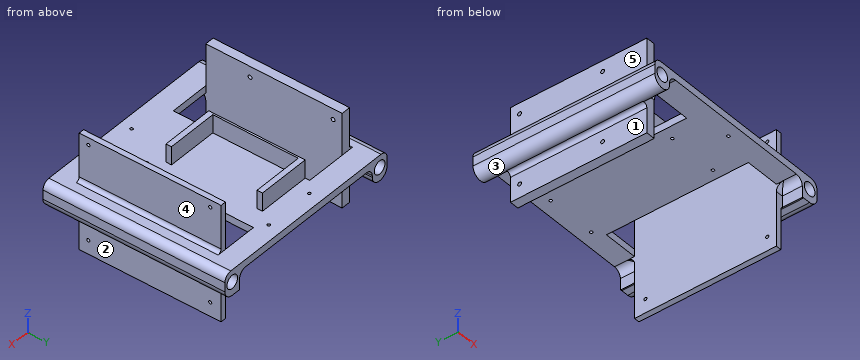
```python
from build123d import *

# Parameters (mm, degrees)
BOSS_EXTRUDE1_DEPTH      = 127
SKETCH3_R                = 4.60374999999995
SKETCH3_R_2              = 4.603749999999996
CUT_EXTRUDE1_DEPTH       = 127
CUT_EXTRUDE10_DEPTH      = 190.225738207042
CUT_EXTRUDE10_DEPTH_BACK = 190.225738207042
SKETCH19_W               = 27.939999999999998
SKETCH19_H               = 99.05999999999997
BOSS_EXTRUDE6_DEPTH      = 3.8099999999999996
CUT_EXTRUDE11_DEPTH      = 183.54455346572246
CUT_EXTRUDE11_DEPTH_BACK = 183.54455346572246
SKETCH23_R               = 1.0999978000000017
SKETCH23_R_2             = 1.0999978000000061
SKETCH23_R_3             = 1.099997799999995
BOSS_EXTRUDE8_DEPTH      = 31.75
BOSS_EXTRUDE8_DEPTH_BACK = 34.29
CUT_EXTRUDE12_DEPTH      = 194.67395901359583
CUT_EXTRUDE12_DEPTH_BACK = 194.67395901359583
CUT_EXTRUDE13_DEPTH      = 194.67395901359583
CUT_EXTRUDE13_DEPTH_BACK = 194.67395901359583
SKETCH32_R               = 0.9999980000000093
SKETCH34_R               = 1.3499972999999863
SKETCH34_R_2             = 1.349997299999995
SKETCH34_R_3             = 1.3499973000000016
CUT_EXTRUDE15_DEPTH      = 15.239999999999998
BOSS_EXTRUDE10_DEPTH     = 12.7
SKETCH36_W               = 1.2700000000000102
SKETCH36_H               = 12.700000000000014
BOSS_EXTRUDE11_DEPTH     = 99.06
FILLET5_R                = 2.54
FILLET6_R                = 2.54
FILLET7_R                = 5.08


with BuildPart() as part:
    # Sketch2 → Boss-Extrude1 (new body)
    with BuildSketch(Plane(origin=(0, 0, 0), x_dir=(1, 0, 0), z_dir=(0, 1, 0))):
        with BuildLine():
            Line((8.7e-16, 11.429999999999996), (8.7e-16, 5.079999999999999))
            ThreePointArc((8.7e-16, 5.079999999999999), (1.4878975515723396, 1.4878975515723383), (5.080000000000001, 0))
            Line((5.080000000000001, 0), (134.61999999999998, 0))
            ThreePointArc((134.61999999999998, 0), (138.21210244842763, 1.4878975515723387), (139.7, 5.08))
            Line((139.7, 5.08), (139.70000000000002, 11.429999999999996))
            ThreePointArc((139.70000000000002, 11.429999999999996), (137.8401280605346, 15.920128060534589), (133.35, 17.78000000000002))
            Line((133.35, 17.78000000000002), (127, 17.780000000000015))
            Line((127, 17.780000000000015), (127, 11.429999999999996))
            Line((127, 11.429999999999996), (127, 5.079999999999999))
            Line((127, 5.079999999999999), (12.699999999999989, 5.08))
            Line((12.699999999999989, 5.08), (12.699999999999989, 11.429999999999996))
            ThreePointArc((12.699999999999989, 11.429999999999996), (6.349999999999994, 17.77999999999999), (8.7e-16, 11.429999999999996))
        make_face()
    extrude(amount=BOSS_EXTRUDE1_DEPTH)

    # Sketch3 → Cut-Extrude1 (cut)
    with BuildSketch(Plane(origin=(0, 127, 0), x_dir=(1, 0, 0), z_dir=(0, 1, 0))):
        with Locations(Location((133.35, 8.41375, 0), (0, 0, 270))):
            Circle(SKETCH3_R)
        with Locations(Location((6.349999999999994, 8.41375, 0), (0, 0, 270))):
            Circle(SKETCH3_R_2)
    extrude(amount=-CUT_EXTRUDE1_DEPTH, mode=Mode.SUBTRACT)

    # Sketch19 → Cut-Extrude10 (cut, two sides: drawn at the far end of the back side and taken through both)
    with BuildSketch(Plane(origin=(4e-17, 0, -5.08), x_dir=(-1, 0, -1e-17), z_dir=(1e-17, 0, -1)).offset(-CUT_EXTRUDE10_DEPTH_BACK)):
        with Locations((-111.76, 63.5)):
            Rectangle(SKETCH19_W, SKETCH19_H)
    extrude(amount=CUT_EXTRUDE10_DEPTH + CUT_EXTRUDE10_DEPTH_BACK, mode=Mode.SUBTRACT)

    # Sketch20 → Boss-Extrude6 (add)
    with BuildSketch(Plane(origin=(125.73, 0, 9.5e-16), x_dir=(1e-17, 0, -1), z_dir=(1, 0, 1e-17))):
        Polygon((5.08, 113.02999999999999), (48.26, 113.02999999999999), (48.26000000000001, 13.97000000000001), (5.08, 13.97000000000001), (-1.06e-15, 13.97000000000001), (-33.01999999999999, 13.97000000000001), (-33.02, 113.02999999999999), (-1.06e-15, 113.02999999999999), align=None)
    extrude(amount=-BOSS_EXTRUDE6_DEPTH)

    # Sketch23 → Cut-Extrude11 (cut, two sides: drawn at the far end of the back side and taken through both)
    with BuildSketch(Plane.ZY.offset(-121.92000000000002).offset(-CUT_EXTRUDE11_DEPTH_BACK)):
        with Locations((27.94, 105.45831715747836)):
            Circle(SKETCH23_R)
        with Locations((27.94, 20.32000000000001)):
            Circle(SKETCH23_R_2)
        with Locations((-38.55999400000001, 20.32000000000001)):
            Circle(SKETCH23_R_3)
        with Locations((-38.55999400000001, 105.45831715747836)):
            Circle(SKETCH23_R_3)
    extrude(amount=CUT_EXTRUDE11_DEPTH + CUT_EXTRUDE11_DEPTH_BACK, mode=Mode.SUBTRACT)

    # Sketch26 → Boss-Extrude8 (add, two sides: drawn at the far end of the back side and taken through both)
    with BuildSketch(Plane(origin=(4e-17, 0, -5.08), x_dir=(-1, 0, -1e-17), z_dir=(1e-17, 0, -1)).offset(-BOSS_EXTRUDE8_DEPTH_BACK)):
        Polygon((-19.049999999999976, 111.125), (-12.699999999999976, 111.125), (-12.699999999999976, 15.875), (-19.049999999999955, 15.875), align=None)
    extrude(amount=BOSS_EXTRUDE8_DEPTH + BOSS_EXTRUDE8_DEPTH_BACK)

    # Sketch27 → Cut-Extrude12 (cut, two sides: drawn at the far end of the back side and taken through both)
    with BuildSketch(Plane(origin=(4e-17, 0, -5.08), x_dir=(-1, 0, -1e-17), z_dir=(1e-17, 0, -1)).offset(-CUT_EXTRUDE12_DEPTH_BACK)):
        Polygon((-19.049999999999976, 15.875), (-46.989999999999974, 15.874999999999996), (-46.989999999999974, 111.125), (-19.049999999999976, 111.125), align=None)
    extrude(amount=CUT_EXTRUDE12_DEPTH + CUT_EXTRUDE12_DEPTH_BACK, mode=Mode.SUBTRACT)

    # Sketch32 → Cut-Extrude13 (cut, two sides: drawn at the far end of the back side and taken through both)
    with BuildSketch(Plane(origin=(4e-17, 0, -5.08), x_dir=(-1, 0, -1e-17), z_dir=(1e-17, 0, -1)).offset(-CUT_EXTRUDE13_DEPTH_BACK)):
        with Locations((-90.80499999999999, 118.02000779999999)):
            Circle(SKETCH32_R)
        with Locations((-55.8049938, 118.02000779999999)):
            Circle(SKETCH32_R)
        with Locations((-55.8049938, 33.02)):
            Circle(SKETCH32_R)
        with Locations((-90.80499999999999, 33.02)):
            Circle(SKETCH32_R)
        with Locations((-73.3049969, 8.019999200000003)):
            Circle(SKETCH32_R)
    extrude(amount=CUT_EXTRUDE13_DEPTH + CUT_EXTRUDE13_DEPTH_BACK, mode=Mode.SUBTRACT)

    # Sketch34 → Cut-Extrude15 (cut)
    with BuildSketch(Plane.ZY.offset(-12.699999999999976)):
        with Locations(Location((-27.30500000000001, 104.775, 0), (0, 0, 270))):
            Circle(SKETCH34_R)
        with Locations(Location((21.695003599999986, 104.775, 0), (0, 0, 270))):
            Circle(SKETCH34_R)
        with Locations(Location((21.695003599999993, 46.774989000000026, 0), (0, 0, 270))):
            Circle(SKETCH34_R_2)
        with Locations(Location((-27.305000000000003, 46.77498900000001, 0), (0, 0, 270))):
            Circle(SKETCH34_R_3)
    extrude(amount=-CUT_EXTRUDE15_DEPTH, mode=Mode.SUBTRACT)

    # Sketch35 → Boss-Extrude10 (add)
    with BuildSketch(Plane.XY):
        Polygon((48.25999999999998, 104.14154915842353), (48.259999999999984, 44.45154915842352), (83.81999999999998, 44.451549158423525), (83.81999999999998, 40.64154915842352), (46.989999999999974, 40.641549158423516), (46.989999999999974, 107.95154915842352), (83.81999999999996, 107.95154915842353), (83.81999999999996, 104.14154915842353), align=None)
    extrude(amount=BOSS_EXTRUDE10_DEPTH)

    # Sketch36 → Boss-Extrude11 (add)
    with BuildSketch(Plane.XZ.offset(-13.97000000000001)):
        with Locations((126.36500000000001, -11.430000000000009)):
            Rectangle(SKETCH36_W, SKETCH36_H)
    extrude(amount=-BOSS_EXTRUDE11_DEPTH)

    # Fillet5
    fillet5_edges = [part.edges().sort_by_distance(p)[0] for p in [
        (12.699999999999989, 63.5, -11.429999999999996),
    ]]
    fillet(fillet5_edges, radius=FILLET5_R)

    # Fillet6
    fillet6_edges = [part.edges().sort_by_distance(p)[0] for p in [
        (125.73, 63.5, 0),
        (12.699999999999976, 63.5, 0),
        (125.73, 63.500000000000014, -17.780000000000015),
    ]]
    fillet(fillet6_edges, radius=FILLET6_R)

    # Fillet7
    fillet7_edges = [part.edges().sort_by_distance(p)[0] for p in [
        (12.699999999999989, 7.9375, -5.08),
        (15.874999999999986, 111.125, -5.08),
        (15.874999999999972, 15.875, -5.08),
        (12.699999999999989, 119.0625, -5.08),
        (127, 120.01500000000001, -5.079999999999999),
        (127, 6.985000000000005, -5.079999999999999),
        (124.46000000000001, 13.97000000000001, -5.08),
        (124.46000000000001, 113.03, -5.08),
    ]]
    fillet(fillet7_edges, radius=FILLET7_R - 0.0001)  # a hair under: the kernel refuses the full size


solid = part.part
```
The listing builds one solid part. Answer for the finished solid, in the listing's coordinates (mm). Face numbers are marked on the shaded views. A direction names the side the tool comes from. Coordinates: 2 decimals unless noted, no trailing zeros. Loops run counter-clockwise (first coordinate to the right, second up) from the corner with the lowest first, then second, coordinate; pieces in that order, holes last. Notation, with made-up numbers: M -10,62 L 48,62 A22 cw 48,78 Z; hole C 26,87.25 d9. An arc over 180 degrees is marked long. Answer as a JSON object with one key per item and string values. Group by question number.
Item 1: Section C-C (z = -43) is taken. Write down the section's boundary in (x, y).
Item 2: Section B-B (y = 86) is taken. Give the number of separate pieces and of enclosed holes in the cut face, and give its area (3 significant figures).
Item 3: Section A-A (x = 112) is taken. Write down the section's boundary in (y, z), and give its area (3 significant figures).
Item 4: Consider L1, parallel to Y at x = 123.45, z = 27.94; L2, parallel to X at y = 75.5, z = -2.5; L3, parallel to X at y = 77.5, z = -36. Determine where each line is inside the solid, lowest interval first.
Item 5: Section D-D (x = 85.5) is taken. Write down the section's boundary in (y, z), and give its area (3 significant figures).
Item 6: Which of the six approach directions +Z, -Z, +X, -X, +Y, -Y give full straight-line access (tool end or side, diameter ignored) to the marked faces 1 and 2?
Item 7: Each of these flat-tipped pins is pushed along its axis until it touches: P1, Ø12, axis at y = 90, z = -32, coming from the -X side; P2, Ø14, axis at y = 80, z = 5, coming from the +X side; P3, Ø4, axis at x = 67.5, z = 8, coming from the -Y side. Where does it stop, or does it pass through?
Item 8: Determine the mould class of the marked faces 3, 4 and 5 for opening direction X: +X half, -X half, draft (parallel to the pull), parting line (faces both ways), or undercut.
Solved:
{
 "1": {"outline": "M 121.92,13.97 L 125.73,13.97 L 125.73,113.03 L 121.92,113.03 Z"},
 "2": {"separate pieces": "3", "enclosed holes": "2", "area": "1,320 mm2"},
 "3": {"outline": "M 0,-5.08 L 13.97,-5.08 L 13.97,0 L 0,0 Z; M 113.03,-5.08 L 127,-5.08 L 127,0 L 113.03,0 Z", "area": "142 mm2"},
 "4": {"L1": "y = 13.97 to 19.22, 21.42 to 104.36, 106.56 to 113.03", "L2": "x = 0.7 to 19.05, 46.99 to 97.79, 121.92 to 139", "L3": "x = 12.7 to 19.05, 121.92 to 125.73"},
 "5": {"outline": "M 0,-5.08 L 127,-5.08 L 127,0 L 0,0 Z", "area": "645 mm2"},
 "6": {"face 1": "-Z, -X, +Y, -Y", "face 2": "-Z, +X, +Y, -Y"},
 "7": {"P1": "stops at x = 12.7", "P2": "stops at x = 138.66", "P3": "stops at y = 40.64"},
 "8": {"face 3": "undercut", "face 4": "+X half", "face 5": "-X half"}
}
